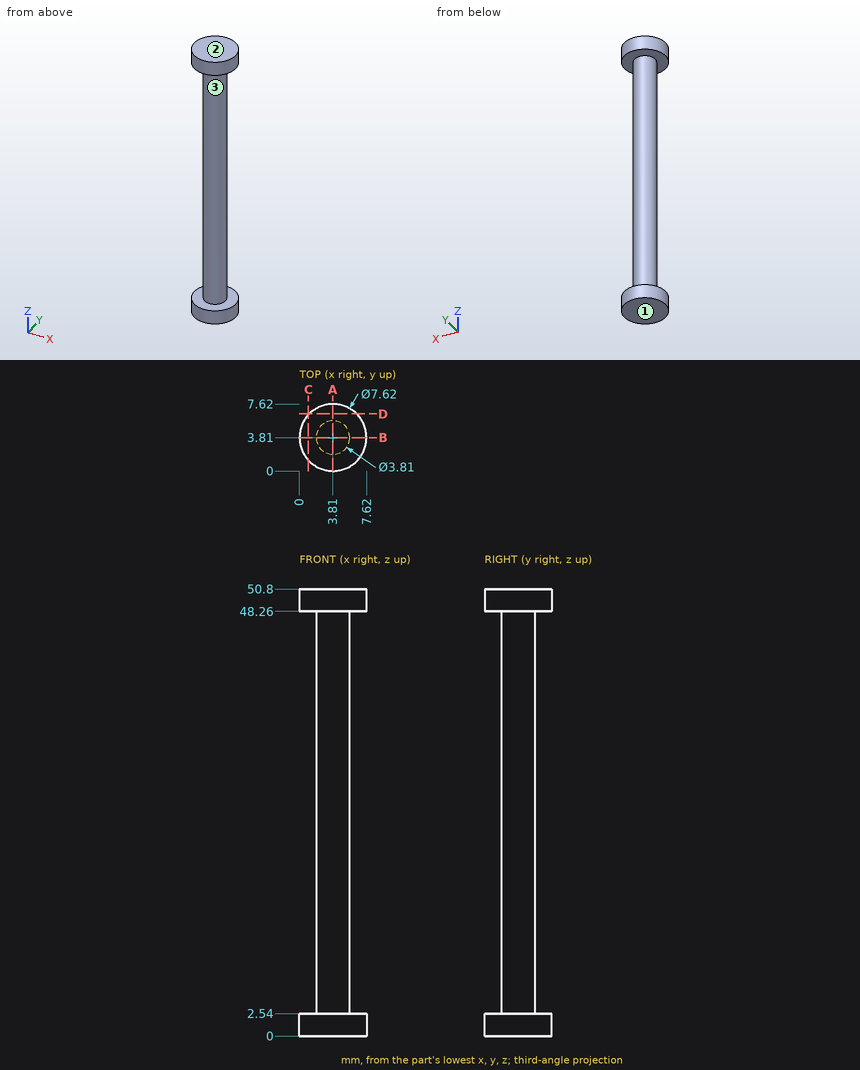
Could you check a few things on this drawing? It's one solid part, dimensions in mm from its lowest x, y, z. Coordinates: 2 decimals unless noted, no trailing zeros. Write each loop counter-clockwise with the first axis right and the second up, starting at its lowest first coordinate (ties: lowest second). Pieces come first, ordered by that corner, then holes.
1) If we section it at A-A (x = 3.81): List the corners of the cut face in (y, z) for me (3 decimals).
Filled in:
outline: (0, 0) - (7.62, 0) - (7.62, 2.54) - (5.715, 2.54) - (5.715, 48.26) - (7.62, 48.26) - (7.62, 50.8) - (0, 50.8) - (0, 48.26) - (1.905, 48.26) - (1.905, 2.54) - (0, 2.54) - close
2) Thinking about a two-plate mould opening in Z: for the marked faces 1, 2 and 3, which applies, +Z half, -Z half, draft (parallel to the pull), parting line (faces both ways), or undercut?
Filled in:
face 1: -Z half
face 2: +Z half
face 3: undercut
3) If we section it at D-D (y = 6.5): List the corners of the cut face in (x, z) for me.
Filled in:
outline: (1.11, 0) - (6.51, 0) - (6.51, 2.54) - (1.11, 2.54) - close; (1.11, 48.26) - (6.51, 48.26) - (6.51, 50.8) - (1.11, 50.8) - close
4) If we section it at C-C (x = 1): List the corners of the cut face in (y, z) for me.
Filled in:
outline: (1.24, 0) - (6.38, 0) - (6.38, 2.54) - (1.24, 2.54) - close; (1.24, 48.26) - (6.38, 48.26) - (6.38, 50.8) - (1.24, 50.8) - close
5) If I drill on line 1 (Z direction, x = 6, y = 2.75); line 2 (X direction, y = 3.75, z = 14.5), over which ranges is the centre line in solid material (lowest first)?
Filled in:
line 1: z = 0 to 2.54, 48.26 to 50.8
line 2: x = 1.91 to 5.71
6) I'm going to push flat-ended pins straight in: pin 1 (4 mm diameter, centred on y = 6, z = 7.5, fed in from -X); pin 2 (4 mm diameter, centred on y = 3.5, z = 33, fed in from +X) (3 decimals); pin 3 (2 mm diameter, centred on x = 4.5, y = 2.5, fed in from -Z); pin 4 (1.5 mm diameter, centred on x = 2, z = 36, fed in from +Y). Where does each tip first touch, or does it pass through?
Filled in:
pin 1: stops at x = 1.91
pin 2: stops at x = 5.715
pin 3: stops at z = 0
pin 4: stops at y = 5.39
